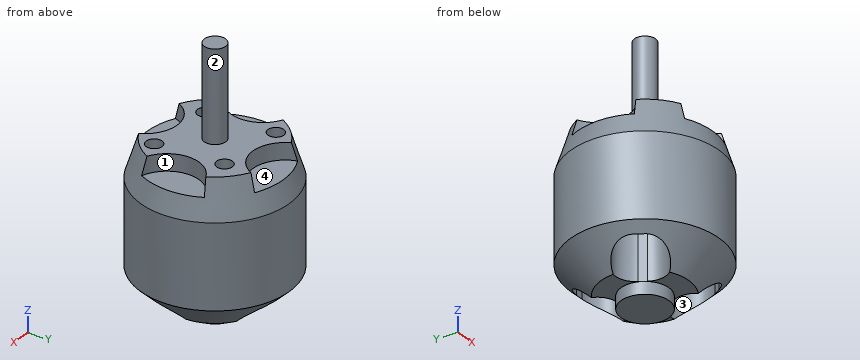
from build123d import *

# Parameters (mm, degrees)
SKETCH1_R           = 13.98905
BOSS_EXTRUDE1_DEPTH = 15.6591
SKETCH2_R           = 11.811
SKETCH4_R           = 8.255
SKETCH5_R           = 4.5085
BOSS_EXTRUDE2_DEPTH = 2.286
CUT_EXTRUDE1_DEPTH  = 9.144
CIRPATTERN1_COUNT   = 3
SKETCH7_R           = 6.075765912
CUT_EXTRUDE2_DEPTH  = 3.1242
CIRPATTERN2_COUNT   = 4
SKETCH8_R           = 2
BOSS_EXTRUDE3_DEPTH = 17
SKETCH9_R           = 1.5
CUT_EXTRUDE3_DEPTH  = 8.11


with BuildPart() as part:
    # Sketch1 → Boss-Extrude1 (new body)
    with BuildSketch(Plane.XY):
        Circle(SKETCH1_R)
    extrude(amount=BOSS_EXTRUDE1_DEPTH)

    # Sketch2 → section 1 of loft1
    with BuildSketch(Plane.XY.offset(22.5806), mode=Mode.PRIVATE) as loft1_s1:
        Circle(SKETCH2_R)
    # loft up to a face of the part (loft1)
    loft([Face(Wire([part.edges().sort_by_distance((-9.576163692, 10.197578577, 15.6591))[0]])), loft1_s1.sketch])

    # Sketch4 → section 1 of loft2
    with BuildSketch(Plane(origin=(0, 0, -5.588), x_dir=(-1, 0, 0), z_dir=(0, 0, -1)), mode=Mode.PRIVATE) as loft2_s1:
        Circle(SKETCH4_R)
    # loft up to a face of the part (loft2)
    loft([Face(Wire([part.edges().sort_by_distance((-9.576163692, -10.197578577, 0))[0]])), loft2_s1.sketch])

    # Sketch5 → Boss-Extrude2 (add)
    with BuildSketch(Plane(origin=(0, 0, -5.588), x_dir=(-1, 0, 0), z_dir=(0, 0, -1))):
        Circle(SKETCH5_R)
    extrude(amount=BOSS_EXTRUDE2_DEPTH)

    # Sketch6 → Cut-Extrude1 (cut)
    with BuildSketch(Plane(origin=(0, 0, -5.588), x_dir=(-1, 0, 0), z_dir=(0, 0, -1))):
        with BuildLine():
            Line((-0.722628041, 12.2555), (0.722628041, 12.2555))
            ThreePointArc((0.722628041, 12.2555), (4.596128041, 8.382), (0.722628041, 4.5085))
            Line((0.722628041, 4.5085), (-0.722628041, 4.5085))
            ThreePointArc((-0.722628041, 4.5085), (-4.596128041, 8.382), (-0.722628041, 12.2555))
        make_face()
    cut_extrude1 = extrude(amount=-CUT_EXTRUDE1_DEPTH, mode=Mode.SUBTRACT)

    # CirPattern1: Cut-Extrude1 ×3 about axis
    cirpattern1_axis = Axis((0, 0, 0), (0, 0, 1))
    for i in range(1, CIRPATTERN1_COUNT):
        add(cut_extrude1.rotate(cirpattern1_axis, i * 360 / CIRPATTERN1_COUNT), mode=Mode.SUBTRACT)

    # Sketch7 → Cut-Extrude2 (cut)
    with BuildSketch(Plane.XY.offset(22.5806)):
        with Locations((0, 13.075508189)):
            Circle(SKETCH7_R)
    cut_extrude2 = extrude(amount=-CUT_EXTRUDE2_DEPTH, mode=Mode.SUBTRACT)

    # CirPattern2: Cut-Extrude2 ×4 about axis
    cirpattern2_axis = Axis((0, 0, 0), (0, 0, 1))
    for i in range(1, CIRPATTERN2_COUNT):
        add(cut_extrude2.rotate(cirpattern2_axis, i * 360 / CIRPATTERN2_COUNT), mode=Mode.SUBTRACT)

    # Sketch8 → Boss-Extrude3 (add)
    with BuildSketch(Plane.XY.offset(22.5806)):
        Circle(SKETCH8_R)
    extrude(amount=BOSS_EXTRUDE3_DEPTH)

    # Sketch9 → Cut-Extrude3 (cut)
    with BuildSketch(Plane.XY.offset(22.5806)):
        with Locations((-6.717514421, 6.717514421)):
            Circle(SKETCH9_R)
        with Locations((6.717514421, -6.717514421)):
            Circle(SKETCH9_R)
        with Locations((5.656854249, 5.656854249)):
            Circle(SKETCH9_R)
        with Locations((-5.656854249, -5.656854249)):
            Circle(SKETCH9_R)
    extrude(amount=-CUT_EXTRUDE3_DEPTH, mode=Mode.SUBTRACT)


solid = part.part
Geometry check sheet. Reference: the model listing, model coordinates, mm. Face numbers are marked on the shaded views. A direction names the side the tool comes from. Give positions to 0.01 mm unless a question says otherwise; leave off trailing zeros. Write each loop counter-clockwise with the first axis right and the second up, starting at its lowest first coordinate (ties: lowest second). Pieces come first, ordered by that corner, then holes. Notation, with made-up numbers: M 15,52 L 24,52 A13 ccw 24,70 Z; hole C -13.75,-40 d8. An arc over 180 degrees is marked long. Answer as CSV lines item,"result". Start each with the question number.
Q1. Section check A-A, the plane z = 32.5. Record the cut outline in (x, y), then the cut area to 3 significant figures.
Q2. Tool access check on the marked faces 1, 2, 3 and 4. Record the directions out of +Z, -Z, +X, -X, +Y, -Y that give a thin tool (end or side, any length) a straight path to the whole face; none if there is none.
Q3. Go/stop test with flat-tipped pins: pin 1 (6 mm diameter, centred on x = -6, z = 30.5, fed in from +Y); pin 2 (6.5 mm diameter, centred on x = -0.5, y = -9, fed in from +Z); pin 3 (1 mm diameter, centred on y = 7.5, z = 4.5, fed in from -X); pin 4 (8 mm diameter, centred on y = 4.5, z = 17, fed in from -X). Record where each tip stops, or that it passes through.
Q4. Section check B-B, the plane z = 9.5. Record the cut outline in (x, y).
Q5. Material ranges on L1, parallel to X at y = -4.75, z = -0.5; L2, parallel to Z at x = 1.5, y = -9.5; L3, parallel to Z at x = 6.5, y = -0.25, recorded low to high.
Geometry says:
1,outline,"C 0,0 d4"
1,area,"12.6 mm^2"
2,face 1,"+Z, +X"
2,face 2,"+Z"
2,face 3,"-Z"
2,face 4,"+Z, +Y"
3,pin 1,"through"
3,pin 2,"z = 22.58"
3,pin 3,"x = -12.11"
3,pin 4,"x = -13.97"
4,outline,"C 0,0 d27.98"
5,L1,"-12.61 to -11.31, -3.02 to 3.02, 11.31 to 12.61"
5,L2,"-4.26 to 19.46"
5,L3,"3.56 to 22.58"
